Read the model definition and answer for the solid it produces. Units are mm, in the model's axes. A direction names the side the tool comes from. Give positions to 0.01 mm unless a question says otherwise; leave off trailing zeros. Loops run counter-clockwise (first coordinate to the right, second up) from the corner with the lowest first, then second, coordinate; pieces in that order, holes last. Notation, with made-up numbers: M 84.5,36 L 120.5,36 A21 ccw 120.5,41 Z; hole C 38.25,68.5 d1. An arc over 180 degrees is marked long. Return JSON: item names as keys, results as strings. Group by question number.
```python
from build123d import *

# Parameters (mm, degrees)
BASE_EXTRUDE_DEPTH      = 15
SKETCH2_R               = 8.331
SKETCH2_R_2             = 7
CUT_EXTRUDE1_DEPTH      = 12
SKETCH4_R               = 6.75
BOSS_EXTRUDE1_DEPTH     = 5
BOSS_EXTRUDE2_START     = 20
BOSS_EXTRUDE2_OUTLINE_R = 10.5
BOSS_EXTRUDE2_DEPTH     = 34
SKETCH6_R               = 8.5
BOSS_EXTRUDE3_DEPTH     = 60
CUT_EXTRUDE3_START      = -60
SKETCH7_R               = 7
CUT_EXTRUDE3_DEPTH      = 60
SKETCH3_R               = 3.5
CUT_EXTRUDE2_DEPTH      = 116.231650745


# Read off the part's stored shape, not the designer's step: Boss-Extrude2
with BuildPart() as part:
    # Sketch1 → Base-Extrude (new body)
    with BuildSketch(Plane.XY):
        Polygon((0, 12.701705922), (-11, 6.350852961), (-11, -6.350852961), (0, -12.701705922), (11, -6.350852961), (11, 6.350852961), align=None)
    extrude(amount=BASE_EXTRUDE_DEPTH)

    # Sketch2 → Cut-Extrude1 (cut)
    with BuildSketch(Plane(origin=(0, 0, 0), x_dir=(-1, 0, 0), z_dir=(0, 0, -1))):
        Circle(SKETCH2_R)
        Circle(SKETCH2_R_2, mode=Mode.SUBTRACT)
    extrude(amount=-CUT_EXTRUDE1_DEPTH, mode=Mode.SUBTRACT)

    # Sketch4 → Boss-Extrude1 (add)
    with BuildSketch(Plane.XY.offset(15)):
        with Locations(Location((0, 0, 0), (0, 0, 180))):
            Circle(SKETCH4_R)
    extrude(amount=BOSS_EXTRUDE1_DEPTH)

    # Boss-Extrude2 outline → Boss-Extrude2 (add)
    with BuildSketch(Plane.XY.offset(BOSS_EXTRUDE2_START)):
        Circle(BOSS_EXTRUDE2_OUTLINE_R)
    extrude(amount=BOSS_EXTRUDE2_DEPTH)

    # Sketch6 → Boss-Extrude3 (add)
    with BuildSketch(Plane.XY.offset(54)):
        Circle(SKETCH6_R)
    extrude(amount=BOSS_EXTRUDE3_DEPTH)

    # Sketch7 → Cut-Extrude3 (cut)
    with BuildSketch(Plane.XY.offset(114).offset(CUT_EXTRUDE3_START)):
        with Locations(Location((0, 0, 0), (0, 0, 180))):
            Circle(SKETCH7_R)
    extrude(amount=CUT_EXTRUDE3_DEPTH, mode=Mode.SUBTRACT)

    # Sketch3 → Cut-Extrude2 (cut, through all)
    with BuildSketch(Plane(origin=(0, 0, 0), x_dir=(-1, 0, 0), z_dir=(0, 0, -1))):
        Circle(SKETCH3_R)
    extrude(amount=-CUT_EXTRUDE2_DEPTH, mode=Mode.SUBTRACT)


solid = part.part
```
1. Flat-ended cylindrical pins translate along their axes: P1, Ø10, axis at x = -2, z = 79.5, coming from the -Y side; P2, Ø1.5, axis at x = -6.5, z = 13, coming from the +Y side; P3, Ø3, axis at x = 5, z = 80.5, coming from the -Y side. Find the tip coordinate at first contact, or state that the pin passes through.
2. Find section D-D (y = 9.5). Write down the section's boundary in (x, z), and give its area (3 significant figures).
3. Find section C-C (z = 29). Write down the section's boundary in (x, y), and give its area (3 significant figures).
4. Find section B-B (z = 70.5). Write down the section's boundary in (x, y).
5. The mould has two halves that part along Y. Classify faces 1 (the flat face through (0, -7, 20)), 2 (the flat face through (-3, 3, 54)), 3 (the cylindrical face through (10, 3.2, 36.8)): +Y half, -Y half, draft (parallel to the pull), parting line (faces both ways), or undercut.
6. Straight lines are drawn through the part: line 1 along Z through (x, y) = (5, 5); line 2 along Y through (x, z) = (0, 72.5); line 3 along Z through (x, y) = (-6.25, -7.75). For each, find the intervals that lie inside material, in ascending order.
7. For faces 4 (the flat face through (2, 7, 12)), 5 (the cylindrical face through (1.46, 6.59, 17.46)), 6 (the cylindrical face through (-6.466, 2.681, 83.58)), determine the directions among +Z, -Z, +X, -X, +Y, -Y from which every point of the face is accessible in a straight line to the end or side of a thin tool.
Result:
{
 "1": {"P1": "stops at y = -8.5", "P2": "stops at y = 9.38", "P3": "stops at y = -7.75"},
 "2": {"outline": "M -5.55,0 L 5.55,0 L 5.55,15 L -5.55,15 Z; M -4.47,20 L 4.47,20 L 4.47,54 L -4.47,54 Z", "area": "470 mm2"},
 "3": {"outline": "C 0,0 d21; hole C 0,0 d7", "area": "308 mm2"},
 "4": {"outline": "C 0,0 d17; hole C 0,0 d14"},
 "5": {"face 1": "draft", "face 2": "undercut", "face 3": "parting line"},
 "6": {"line 1": "z = 12 to 15, 20 to 114", "line 2": "y = -8.5 to -7, 7 to 8.5", "line 3": "z = 0 to 15, 20 to 54"},
 "7": {"face 4": "-Z", "face 5": "none", "face 6": "+Z"}
}
